Check sheet for the modelled part. Datum: model origin and axes. Units: mm. Face numbers are marked on the shaded views. A direction names the side the tool comes from. Coordinates: 2 decimals unless noted, no trailing zeros. Loops run counter-clockwise (first coordinate to the right, second up) from the corner with the lowest first, then second, coordinate; pieces in that order, holes last. Notation, with made-up numbers: M -20.75,34.5 L -2.75,34.5 A15 cw -2.75,50.5 Z; hole C -39.75,61.25 d9. An arc over 180 degrees is marked long. Use CSV: the item, a comma, the result in double quotes. Start each with the question number.
(1) Section check D-D on x = -12.5. Record the cut outline in (y, z), and give its area (3 significant figures).
(2) Section check A-A on y = 3. Record the cut outline in (x, z).
(3) Scan lines: line 1 (X direction, y = 5, z = 94); line 2 (Z direction, x = 11, y = 4); line 3 (Z direction, x = 11, y = 6). Record each from-to range of solid material in increasing order.
(4) Draft check along Z on the marked faces 4, 5 and 6. Enter one of: pulls with the +Z half, pulls with the -Z half, needs draft (parallel to the pull), parting line crosses it, or undercut.
(5) Set-up check for the marked faces 1, 2 and 3: record each of +Z, -Z, +X, -X, +Y, -Y from which the full face is reachable in a straight line by a thin tool's end or side.
(6) Go/stop test with flat-tipped pins: pin 1 Ø1.5 at (x, z) = (9, 46) entering from -Y; pin 2 Ø8.5 at (x, y) = (-4.5, 24) entering from +Z; pin 3 Ø5 at (x, z) = (-3.5, 16) entering from +Y. Record where each tip stops, or that it passes through.
(7) Section check B-B on z = 51. Record the cut outline in (x, y).
(8) Section check C-C on y = 33.5. Record the cut outline in (x, z), and give its area (3 significant figures).
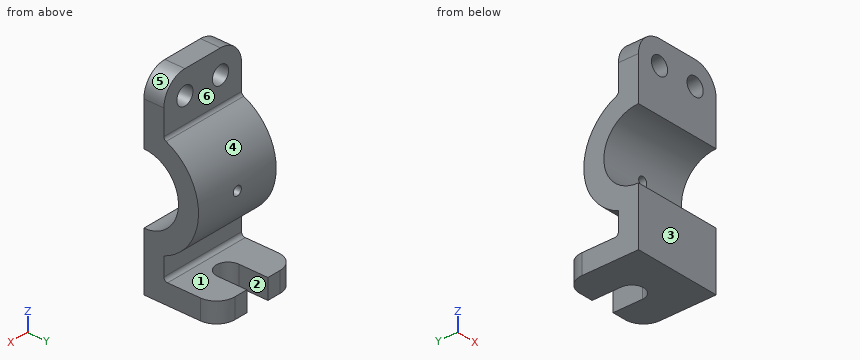
Autodesk Inventor part; units mm, degrees
ref_plane "YZ Plane" through (0, 0, 0) normal (1, 0, 0) x (0, 1, 0)
ref_plane "XZ Plane" through (0, 0, 0) normal (0, 1, 0) x (-1, 0, 0)
ref_plane "XY Plane" through (0, 0, 0) normal (0, 0, 1) x (1, 0, 0)
sketch "Sketch1" plane through (0, 0, 0) normal (1, 0, 0) x (0, 1, 0)
  line L0 (0, 0) -> (41, 0)
  line L1 (0, 0) -> (0, 32)
  arc A0 (0, 32) -> (0, 70) centre (0, 51) ccw
  line L2 (0, 70) -> (0, 107)
  line L3 (41, 11) -> (11, 11)
  line L4 (11, 11) -> (11, 23.0894)
  arc A1 (11, 23.0894) -> (11, 78.9106) centre (0, 51) ccw
  line L5 (11, 78.9106) -> (11, 107)
  line L6 (11, 107) -> (0, 107)
  line L7 (41, 11) -> (41, 0)
  dimension "d0" = 41
  dimension "d1" = 107
  dimension "d2" = 51
  dimension "d3" = 11
  dimension "d4" = 30
extrude "Extrusion1" add sketch "Sketch1" along normal mid plane 48
fillet "Fillet1" radius 13 2 edges at (-24, 5.5, 107) (24, 5.5, 107)
fillet "Fillet2" radius 2 2 edges at (0, 11, 78.9106) (0, 11, 11)
sketch "Sketch2" plane through (-11, 11, 107) normal (0, 1, 0) x (1, 0, 0)
  arc A0 (-13, 13) -> (0, 0) centre (0, 13) ccw
  circle A1 centre (0, 13) radius 5
  arc A2 (22, 0) -> (35, 13) centre (22, 13) ccw
  circle A3 centre (22, 13) radius 5
  point P0 (11, 107)
  dimension "d9" = 10
  dimension "d10" = 10
extrude "Extrusion2" cut sketch "Sketch2" against normal through all
sketch "Sketch3" plane through (24, 41, 0) normal (0, 0, -1) x (-1, 0, 0)
  line L0 (48, 0) -> (0, 0)
  line L1 (30.5, 0) -> (17.5, 0)
  line L2 (17.5, 0) -> (17.5, -16)
  line L3 (30.5, -16) -> (30.5, 0)
  arc A0 (17.5, -16) -> (30.5, -16) centre (24, -16) ccw
  point P0 (24, -41)
  dimension "d14" = 13
  dimension "d17" = 16
  dimension "d18" = 16
extrude "Extrusion3" cut sketch "Sketch3" against normal up to next
fillet "Fillet3" radius 10 2 edges at (-24, 41, 5.5) (24, 41, 5.5)
sketch "Sketch4" plane through (-24, 0, 0) normal (0, -1, 0) x (1, 0, 0)
  line L0 (48, 70) -> (48, 32)
  line L1 (48, 51) -> (0, 51) construction
  line L2 (0, 32) -> (0, 70)
  circle A0 centre (24, 51) radius 2.5
  point P0 (24, 0)
  dimension "d22" = 5
extrude "Extrusion4" cut sketch "Sketch4" against normal through all
thread "Thread1"
properties part number "T05"
Outcome:
1,outline,"M 0,0 L 41,0 L 41,11 L 13,11 A2 cw 11,13 L 11,23.09 A30 ccw 12.19,78.41 A2 cw 11,80.24 L 11,89.23 L 0,89.23 L 0,70 A19 cw 0,32 Z; M 0,98.77 L 11,98.77 L 11,106.91 L 0,106.91 Z"
1,area,"1,600 mm²"
2,outline,"M -24,0 L 24,0 L 24,32.24 L -24,32.24 Z; M -24,69.76 L 24,69.76 L 24,94 A13 ccw 11,107 L -11,107 A13 ccw -24,94 Z; hole C -11,94 d10; hole C 11,94 d10"
3,line 1,"x = -24 to -16, -6 to 6, 16 to 24"
3,line 2,"z = 0 to 32.43, 69.57 to 89, 99 to 107"
3,line 3,"z = 0 to 32.97, 69.03 to 89, 99 to 107"
4,face 4,"undercut"
4,face 5,"pulls with the +Z half"
4,face 6,"needs draft"
5,face 1,"+X, -X, +Y"
5,face 2,"-Z, +Y"
5,face 3,"+Z, -Z, +X, -X, -Y"
6,pin 1,"stops at y = 18.11"
6,pin 2,"stops at z = 73.58"
6,pin 3,"stops at y = 11"
7,outline,"M -24,19 L -2.5,19 L -2.5,30 L -24,30 Z; M 2.5,19 L 24,19 L 24,30 L 2.5,30 Z"
8,outline,"M -23.68,0 L -6.5,0 L -6.5,11 L -23.68,11 Z; M 6.5,0 L 23.68,0 L 23.68,11 L 6.5,11 Z"
8,area,"378 mm²"
